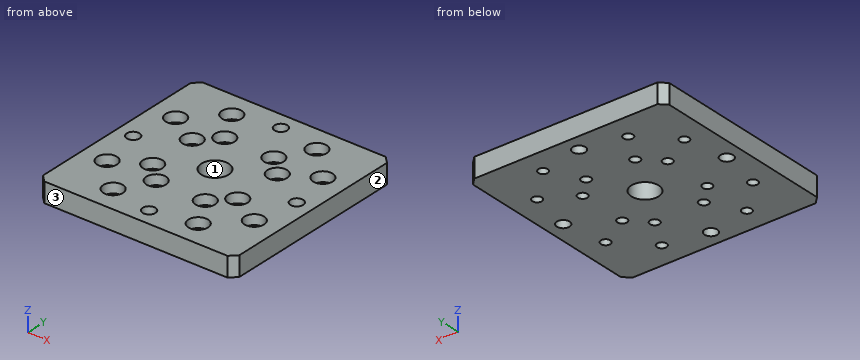
Autodesk Inventor part; units mm, degrees
ref_plane "YZ Plane" through (0, 0, 0) normal (1, 0, 0) x (0, 1, 0)
ref_plane "XZ Plane" through (0, 0, 0) normal (0, 1, 0) x (-1, 0, 0)
ref_plane "XY Plane" through (0, 0, 0) normal (0, 0, 1) x (1, 0, 0)
ref_plane "Work Plane1" through (0, 0, 0) normal (0, 0, 1) x (1, 0, 0)
sketch "Sketch1" plane through (0, 0, 0) normal (0, 0, 1) x (1, 0, 0)
  line L0 (-28, 30) -> (-30, 28)
  line L1 (-30, 28) -> (-30, -28)
  line L2 (-30, -28) -> (-28, -30)
  line L3 (-28, -30) -> (28, -30)
  line L4 (28, -30) -> (30, -28)
  line L5 (30, -28) -> (30, -17.7934)
  line L6 (30, 28) -> (28, 30)
  line L7 (28, 30) -> (17.7934, 30)
  line L8 (-25, -25) -> (25, -25) construction
  line L9 (25, -25) -> (25, 25) construction
  line L10 (25, 25) -> (-25, 25) construction
  line L11 (-25, 25) -> (-25, -25) construction
  line L12 (-25, -25) -> (25, 25) construction
  line L13 (25, -25) -> (-25, 25) construction
  line L14 (30, -17.7934) -> (44, -17.7934)
  line L15 (44, -9.0511) -> (44, -17.7934)
  line L16 (30, -9.0511) -> (44, -9.0511) construction
  line L17 (30, -9.0511) -> (30, 8.3051)
  line L18 (30, 8.3051) -> (44, 8.3051)
  line L19 (44, 19.2331) -> (44, 8.3051)
  line L20 (30, 19.2331) -> (44, 19.2331) construction
  line L21 (30, 28) -> (30, -28)
  line L22 (17.7934, 30) -> (17.7934, 44)
  line L23 (9.0511, 44) -> (17.7934, 44)
  line L24 (9.0511, 30) -> (9.0511, 44) construction
  line L25 (-8.3051, 30) -> (-8.3051, 44)
  line L26 (-19.2331, 44) -> (-8.3051, 44)
  line L27 (-19.2331, 30) -> (-19.2331, 44) construction
  line L28 (-19.2331, 30) -> (-28, 30)
  line L29 (30, 19.2331) -> (30, 28)
  line L30 (9.0511, 30) -> (-8.3051, 30)
  line L31 (-28, 30) -> (28, 30)
  line L32 (25, 0) -> (-25, 0)
  point P0 (0, 0)
  dimension "d0" = 50
  dimension "d1" = 50
extrude "Extrusion1" add sketch "Sketch1" along normal blind 6
sketch "Sketch2" plane through (0, 0, 6) normal (0, 0, 1) x (1, 0, 0)
  line L0 (-25, -25) -> (25, -25)
  line L1 (25, -25) -> (25, 25)
  line L2 (25, 25) -> (-25, 25)
  line L3 (-25, 25) -> (-25, -25)
  line L4 (-25, -25) -> (25, 25) construction
  line L5 (25, -25) -> (-25, 25) construction
  point P0 (0, 0)
  point P1 (25, 0)
  point P2 (-25, 0)
  point P3 (0, 25)
  point P4 (0, -25)
  dimension "d4" = 50
  dimension "d5" = 50
hole "Hole1" at (-25, 0, 6) at (25, 0, 6) direction (0, 0, -1) diameter 3.9 depth 10 tip angle 118
sketch "Sketch3" plane through (0, 0, 6) normal (0, 0, 1) x (1, 0, 0)
  circle A0 centre (25, 0) radius 1.95
  circle A1 centre (-25, 0) radius 1.95
  line L0 (-28, 30) -> (-30, 28)
  line L1 (-30, 28) -> (-30, -28)
  line L2 (-30, -28) -> (-28, -30)
  line L3 (-28, -30) -> (28, -30)
  line L4 (28, -30) -> (30, -28)
  line L5 (30, -28) -> (30, 28)
  line L6 (30, 28) -> (28, 30)
  line L7 (28, 30) -> (-28, 30)
  line L8 (-22.5, -13) -> (22.5, -13) construction
  line L9 (22.5, -13) -> (22.5, 13) construction
  line L10 (22.5, 13) -> (-22.5, 13) construction
  line L11 (-22.5, 13) -> (-22.5, -13) construction
  line L12 (-22.5, -13) -> (22.5, 13) construction
  line L13 (22.5, -13) -> (-22.5, 13) construction
  line L14 (7.5, -13) -> (-7.5, -13) construction
  line L15 (-7.5, -13) -> (-7.5, 13) construction
  line L16 (-7.5, 13) -> (7.5, 13) construction
  line L17 (7.5, 13) -> (7.5, -13) construction
  line L18 (7.5, -13) -> (-7.5, 13) construction
  line L19 (-7.5, -13) -> (7.5, 13) construction
  point P0 (0, 0)
  dimension "d13" = 45
  dimension "d14" = 26
  dimension "d15" = 15
hole "Hole2" at (22.5, 13, 6) at (7.5, 13, 6) at (-7.5, 13, 6) at (-22.5, 13, 6) at (-22.5, -13, 6) at (-7.5, -13, 6) at (7.5, -13, 6) at (22.5, -13, 6) direction (0, 0, -1) diameter 2.9 depth 10 tip angle 118 counterbore diameter 6 counterbore depth 3
sketch "Sketch4" plane through (0, 0, 6) normal (0, 0, 1) x (1, 0, 0)
  circle A0 centre (0, 0) radius 4.1656
pattern_circular "Circular Pattern1" count 2 over 90 about axis through (0, 0, 6) along (0, 0, 1) of "Hole1", "Hole2"
extrude "Extrusion2" cut sketch "Sketch4" against normal blind 10
properties part number "00_XY_stage-CHUO_SEIKI_LD-647-R1-Bottom"
Geometry check sheet. Reference: the model listing, model coordinates, mm. Face numbers are marked on the shaded views. Coordinates: 2 decimals unless noted, no trailing zeros. Order: outer loops, then holes, each group sorted by start corner. A loop starts at its lowest first (then second) coordinate and runs counter-clockwise, first axis right, second up. Notation, with made-up numbers: (22, 36.5) - (76, 36.5) arc R22 cw to (76, 65.5) - close; hole circle Ø2 at (38, -34). An arc over 180 degrees is marked (long way). One line per item, written item: value.
(1) Sectioned sample at D-D (z = 1.1). Count the separate pieces of the cut face and the enclosed holes in it, and give its area (3 significant figures).
Data:
separate pieces: 1
enclosed holes: 21
area: 3,380 mm^2
(2) Sectioned sample at B-B (x = 0). Enter the section's corners in (y, z), and give its area (3 significant figures).
Data:
outline: (-30, 0) - (-26.95, 0) - (-26.95, 6) - (-30, 6) - close; (-23.05, 0) - (-4.17, 0) - (-4.17, 6) - (-23.05, 6) - close; (4.17, 0) - (23.05, 0) - (23.05, 6) - (4.17, 6) - close; (26.95, 0) - (30, 0) - (30, 6) - (26.95, 6) - close
area: 263 mm^2
(3) Depth check by flat-ended pin: pin 1 Ø1.8 at (x, y) = (8.5, -14.5) entering from +Z. Enter the tip coordinate at first touch or a pass-through.
Data:
pin 1: stops at z = 3
(4) Sectioned sample at A-A (y = 7.5). Enter the section's corners in (x, z), and give its area (3 significant figures).
Data:
outline: (-30, 0) - (-14.45, 0) - (-14.45, 3) - (-16, 3) - (-16, 6) - (-30, 6) - close; (-11.55, 0) - (11.55, 0) - (11.55, 3) - (10, 3) - (10, 6) - (-10, 6) - (-10, 3) - (-11.55, 3) - close; (14.45, 0) - (30, 0) - (30, 6) - (16, 6) - (16, 3) - (14.45, 3) - close
area: 307 mm^2
(5) Release check for a two-part mould opening along X. For the marked faces 1, 2 and 3 record: +X half, -X half, draft (parallel to the pull), parting line (faces both ways), or undercut.
Data:
face 1: undercut
face 2: +X half
face 3: draft
(6) Thickness scan on probe 1 along Y at (x, z) = (13, 3.8); probe 2 along Y at (x, z) = (-7.5, 2.05). Record the ranges inside material, lowest first. Write a range as from..to.
Data:
probe 1: y = -30..-25.5, -19.5..-10.5, -4.5..4.5, 10.5..19.5, 25.5..30
probe 2: y = -30..-14.45, -11.55..11.55, 14.45..30
